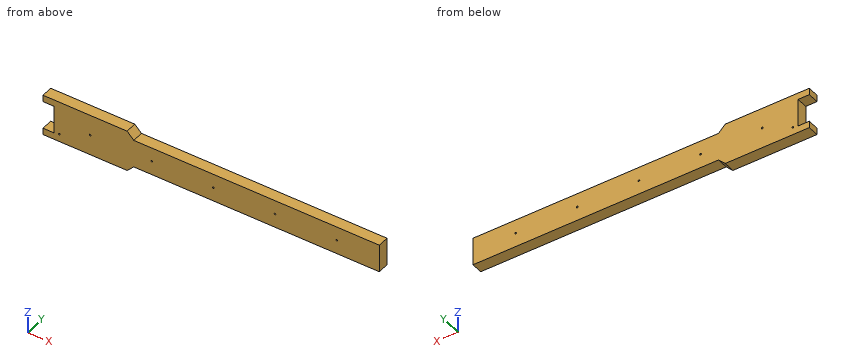
```python
from build123d import *

# Parameters (mm, degrees)
EXTRUDE_1_DEPTH        = 10
SKETCH_2_R             = 0.75
CUT_EXTRUDE_1_DEPTH    = 302.763152157
PATTERN_LINEAR_1_COUNT = 5
PATTERN_LINEAR_1_PITCH = 55
OTHER_1_OUTLINE_R      = 0.75
OTHER_1_DEPTH          = 10


# Read off the part's stored shape, not the designer's step: Отверстие1
with BuildPart() as part:
    # Эскиз1 → Бобышка-Вытянуть1 (new body)
    with BuildSketch(Plane(origin=(0, 0, 0), x_dir=(1, 0, 0), z_dir=(0, 1, 0))):
        Polygon((0, 31), (75, 31), (81, 25), (300, 25), (300, 0), (81, 0), (75, -6), (0, -6), (0, 0), (10, 0), (10, 25), (0, 25), align=None)
    extrude(amount=EXTRUDE_1_DEPTH)

    # Эскиз2 → Вырез-Вытянуть1 (cut, through all)
    with BuildSketch(Plane(origin=(0, 10, 0), x_dir=(1, 0, 0), z_dir=(0, 1, 0))):
        with Locations(Location((42, 12.5, 0), (0, 0, 270))):
            Circle(SKETCH_2_R)
    cut_extrude_1 = extrude(amount=-CUT_EXTRUDE_1_DEPTH, mode=Mode.SUBTRACT)

    # Линейный массив1: Вырез-Вытянуть1 ×5
    with Locations(*[(i * PATTERN_LINEAR_1_PITCH, 0, 0) for i in range(1, PATTERN_LINEAR_1_COUNT)]):
        add(cut_extrude_1, mode=Mode.SUBTRACT)

    # Отверстие1 outline → Отверстие1 (cut)
    with BuildSketch(Plane(origin=(0, 0, 0), x_dir=(1, 0, 0), z_dir=(0, 1, 0))):
        with Locations((14.633333886, 24.136000106)):
            Circle(OTHER_1_OUTLINE_R)
    extrude(amount=OTHER_1_DEPTH, mode=Mode.SUBTRACT)


solid = part.part
```
The model under review builds one solid part; all positions refer to its coordinate system, in mm. Coordinates: 2 decimals unless noted, no trailing zeros. Write each loop counter-clockwise with the first axis right and the second up, starting at its lowest first coordinate (ties: lowest second). Pieces come first, ordered by that corner, then holes. Notation, with made-up numbers: (60.25, -19.5) - (102.25, -19.5) arc R20 cw to (102.25, 6.5) - close; hole circle Ø10 at (-8.5, -28.75). An arc over 180 degrees is marked (long way). Answer in a Markdown table with one row per item. Add a question column.
Q1. Consider section B-B on x = 157.5. Give the boundary of the cut face in (y, z), then the cut area to 3 significant figures.
Q2. Consider section C-C on z = 2.5. Give the boundary of the cut face in (x, y), then the cut area to 3 significant figures.
Q3. Consider section A-A on y = 4.75. Give the boundary of the cut face in (x, z).
Q4. To check wall thickness, follow line 1 along X through (y, z) = (4.5, -12.5); line 2 along Z through (x, y) = (262, 3.5); line 3 along X through (y, z) = (1.25, -23). State the ranges of each line that lie inside material, in increasing order. Write a range as from..to.
Q5. Clearance check with flat-ended pins moving along their axes: pin 1 (3 mm diameter, centred on x = 144, y = 8, fed in from +Z); pin 2 (1.5 mm diameter, centred on x = 226.5, y = 2, fed in from -Z); pin 3 (3 mm diameter, centred on y = 3, z = -8, fed in from -X). State where each tip first meets the part, or that it passes through.
Answers below:
| question | item | result |
|---|---|---|
| 1 | outline | (0, -25) - (10, -25) - (10, 0) - (0, 0) - close |
| 1 | area | 250 mm² |
| 2 | outline | (0, 0) - (78.5, 0) - (78.5, 10) - (0, 10) - close |
| 2 | area | 785 mm² |
| 3 | outline | (0, -31) - (75, -31) - (81, -25) - (300, -25) - (300, 0) - (81, 0) - (75, 6) - (0, 6) - (0, 0) - (10, 0) - (10, -25) - (0, -25) - close; hole circle Ø1.5 at (14.63, -24.14); hole circle Ø1.5 at (42, -12.5); hole circle Ø1.5 at (97, -12.5); hole circle Ø1.5 at (152, -12.5); hole circle Ø1.5 at (207, -12.5); hole circle Ø1.5 at (262, -12.5) |
| 4 | line 1 | 10..41.25, 42.75..96.25, 97.75..151.25, 152.75..206.25, 207.75..261.25, 262.75..300 |
| 4 | line 2 | -25..-13.25, -11.75..0 |
| 4 | line 3 | 10..300 |
| 5 | pin 1 | z = 0 |
| 5 | pin 2 | z = -25 |
| 5 | pin 3 | x = 10 |
